Build history of the part. All positions in model axes, mm. Face numbers are marked on the shaded views. A direction names the side the tool comes from. Round coordinates to 2 decimals unless told otherwise and drop trailing zeros. Order: outer loops, then holes, each group sorted by start corner. A loop starts at its lowest first (then second) coordinate and runs counter-clockwise, first axis right, second up. Notation, with made-up numbers: M -38.75,82.5 L -12.75,82.5 A19 ccw -12.75,99.5 Z; hole C 30.25,21.5 d11. An arc over 180 degrees is marked long. One line per item, written item: value. Start each with the question number.
Item 1: Band-saw the part on B-B, the plane x = 67.5. Write the cut outline in (y, z).
Item 2: Band-saw the part on A-A, the plane z = 24. Write the cut outline in (x, y).
Item 3: Tool access for the marked faces 1 and 2: list every direction of +Z, -Z, +X, -X, +Y, -Y with a clear straight run to the whole face (end or side of a thin tool).
Item 4: Pin check, flat tips, straight feed: pin 1 (5 mm diameter, centred on y = 278, z = 16, fed in from -X); pin 2 (8 mm diameter, centred on y = 279, z = 27.5, fed in from -X); pin 3 (5 mm diameter, centred on x = -244.3, y = 289.2, fed in from +Z); pin 4 (4 mm diameter, centred on x = -182, z = 25.5, fed in from -Y). Stop position of each tip, or through.
Item 5: Probe L1, parallel to X at y = 287.25, z = 5; L2, parallel to X at y = 287.75, z = 34; L3, parallel to Y at x = 96.13, z = 26.5. List the from-to ranges inside material, lowest first.
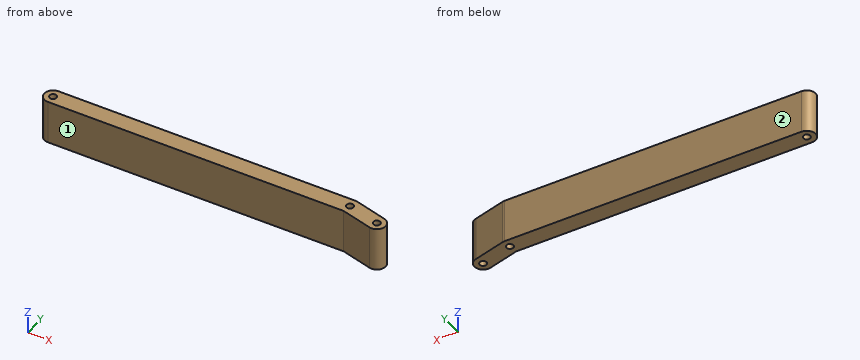
```python
from build123d import *

# Parameters (mm, degrees)
SKETCH1_R           = 4
BOSS_EXTRUDE1_DEPTH = 50


with BuildPart() as part:
    # Sketch1 → Boss-Extrude1 (new body)
    with BuildSketch(Plane.XY):
        with BuildLine():
            Line((94.813332526, 279.2), (130.111538956, 269.740814246))
            ThreePointArc((130.111538956, 269.740814246), (142.359185754, 276.811538956), (135.288461044, 289.059185754))
            Line((135.288461044, 289.059185754), (98.718461044, 298.859185754))
            ThreePointArc((98.718461044, 298.859185754), (97.435400794, 299.11443033), (96.13, 299.2))
            Line((96.13, 299.2), (-244.3, 299.2))
            ThreePointArc((-244.3, 299.2), (-254.3, 289.2), (-244.3, 279.2))
            Line((-244.3, 279.2), (94.813332526, 279.2))
        make_face()
        with Locations((96.13, 289.2)):
            Circle(SKETCH1_R, mode=Mode.SUBTRACT)
        with Locations((132.7, 279.4)):
            Circle(SKETCH1_R, mode=Mode.SUBTRACT)
        with Locations((-244.3, 289.2)):
            Circle(SKETCH1_R, mode=Mode.SUBTRACT)
    extrude(amount=BOSS_EXTRUDE1_DEPTH)


solid = part.part
```
Output:
1. outline: M 279.2,0 L 299.2,0 L 299.2,50 L 279.2,50 Z
2. outline: M -244.3,279.2 L 94.81,279.2 L 130.11,269.74 A10 ccw 135.29,289.06 L 98.72,298.86 A10 ccw 96.13,299.2 L -244.3,299.2 A10 ccw Z; hole C -244.3,289.2 d8; hole C 96.13,289.2 d8; hole C 132.7,279.4 d8
3. face 1: +Z, -Z, -X, -Y
3. face 2: +Z, -Z, +X, -X, +Y
4. pin 1: stops at x = -249.23
4. pin 2: stops at x = -252.15
4. pin 3: passes through
4. pin 4: stops at y = 279.2
5. L1: x = -254.11 to -247.79, -240.81 to 92.64, 99.62 to 138.89
5. L2: x = -254.19 to -248.03, -240.57 to 92.4, 99.86 to 138.2
5. L3: y = 278.85 to 285.2, 293.2 to 299.2
